Design review of the part built by this model. Coordinates are the model's own, in mm. Face numbers are marked on the shaded views. A direction names the side the tool comes from. Give positions to 0.01 mm unless a question says otherwise; leave off trailing zeros. Write each loop counter-clockwise with the first axis right and the second up, starting at its lowest first coordinate (ties: lowest second). Pieces come first, ordered by that corner, then holes.
```python
from build123d import *

# Parameters (mm, degrees)
SKETCH1_W             = 23
SKETCH1_H             = 53.06
SKETCH1_R             = 1.4732
SKETCH1_H_2           = 3.175
BOSS_EXTRUDE1_DEPTH   = 3.175
BOSS_EXTRUDE2_START   = 3.175
SKETCH1_3_W           = 23
SKETCH1_3_H           = 3.175
BOSS_EXTRUDE2_DEPTH   = 9
F_8_32_TAPPED_HOLE1_D = 3.4544
FILLET1_R             = 1


with BuildPart() as part:
    # Sketch1 → Boss-Extrude1 (new body)
    # profile 1 of 2: a face of its own
    with BuildSketch(Plane.XY):
        with Locations((11.5, -26.53)):
            Rectangle(SKETCH1_W, SKETCH1_H)
        with Locations((2.5, -5.5)):
            Circle(SKETCH1_R, mode=Mode.SUBTRACT)
        with Locations((20.5, -5.5)):
            Circle(SKETCH1_R, mode=Mode.SUBTRACT)
    # profile 2 of 2: a face of its own
    with BuildSketch(Plane.XY):
        with Locations((11.5, -54.6475)):
            Rectangle(SKETCH1_W, SKETCH1_H_2)
    extrude(amount=BOSS_EXTRUDE1_DEPTH)

    # Sketch1<3> → Boss-Extrude2 (add)
    with BuildSketch(Plane.XY.offset(BOSS_EXTRUDE2_START)):
        with Locations((11.5, -54.6475)):
            Rectangle(SKETCH1_3_W, SKETCH1_3_H)
    extrude(amount=BOSS_EXTRUDE2_DEPTH)

    # #8-32 Tapped Hole1 (through all)
    with Locations(Plane(origin=(11.5, -53.06, 8.175), x_dir=(0, 0, 1), z_dir=(0, 1, 0))):
        with Locations((0, 0)):
            Hole(F_8_32_TAPPED_HOLE1_D / 2)

    # Fillet1
    fillet1_edges = [part.edges().sort_by_distance(p)[0] for p in [
        (0, 0, 1.5875),
        (23, 0, 1.5875),
        (0, -54.6475, 12.175),
        (11.5, -53.06, 3.175),
        (23, -54.6475, 12.175),
        (11.5, -56.235, 0),
    ]]
    fillet(fillet1_edges, radius=FILLET1_R)


solid = part.part
```
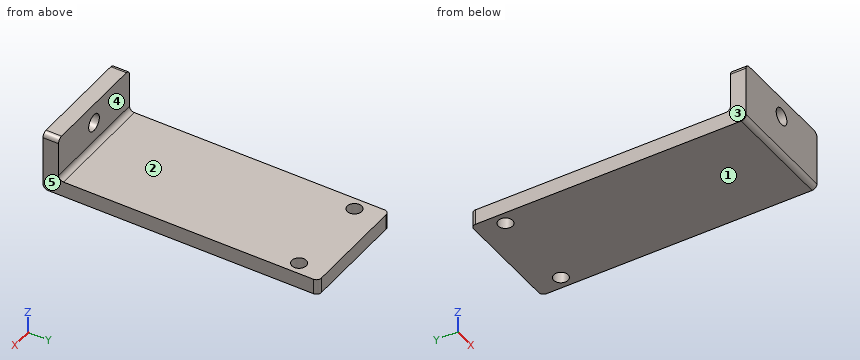
(1) To check wall thickness, follow L1, parallel to Y at x = 20.5, z = 0.9; L2, parallel to Z at x = 9.5, y = -17 (3 decimals); L3, parallel to Y at x = 4.25, z = 7.5 (3 decimals). State the ranges of each line that lie inside material, in increasing order.
Resolved:
L1: y = -56.23 to -6.97, -4.03 to 0
L2: z = 0 to 3.175
L3: y = -56.235 to -53.06
(2) Consider section A-A, the plane x = 2.5. Give the boundary of the cut face in (y, z) (3 decimals).
Resolved:
outline: (-56.235, 1) arc R1 ccw to (-55.235, 0) - (-6.973, 0) - (-6.973, 3.175) - (-52.06, 3.175) arc R1 cw to (-53.06, 4.175) - (-53.06, 12.175) - (-56.235, 12.175) - close; (-4.027, 0) - (0, 0) - (0, 3.175) - (-4.027, 3.175) - close
(3) Consider section B-B, the plane y = -5.5. Give the boundary of the cut face in (x, z) (3 decimals), then the cut area to 3 significant figures.
Resolved:
outline: (0, 0) - (1.027, 0) - (1.027, 3.175) - (0, 3.175) - close; (3.973, 0) - (19.027, 0) - (19.027, 3.175) - (3.973, 3.175) - close; (21.973, 0) - (23, 0) - (23, 3.175) - (21.973, 3.175) - close
area: 54.3 mm2
(4) Consider section D-D, the plane x = 14. Give the boundary of the cut face in (y, z) (3 decimals), then the cut area to 3 significant figures.
Resolved:
outline: (-56.235, 1) arc R1 ccw to (-55.235, 0) - (0, 0) - (0, 3.175) - (-52.06, 3.175) arc R1 cw to (-53.06, 4.175) - (-53.06, 12.175) - (-56.235, 12.175) - close
area: 207 mm2
(5) Mouldability with a two-part tool opening along Z and no side actions: class the marked faces 1, 2 and 3 as pulls with the +Z half, pulls with the -Z half, needs draft (parallel to the pull), parting line crosses it, or undercut.
Resolved:
face 1: pulls with the -Z half
face 2: pulls with the +Z half
face 3: needs draft
(6) Clearance check with flat-ended pins moving along their axes: P1, Ø1, axis at y = -23.5, z = 5, coming from the -X side; P2, Ø3, axis at x = 8.5, y = -14.5, coming from the +Z side (3 decimals). State where each tip first meets the part, or that it passes through.
Resolved:
P1: passes through
P2: stops at z = 3.175
(7) Consider section C-C, the plane z = 8. Give the boundary of the cut face in (x, y) (3 decimals), then the cut area to 3 significant figures.
Resolved:
outline: (0, -56.235) - (9.782, -56.235) - (9.782, -53.06) - (0, -53.06) - close; (13.218, -56.235) - (23, -56.235) - (23, -53.06) - (13.218, -53.06) - close
area: 62.1 mm2
(8) Tool access review of the marked faces 4 and 5: name each direction out of +Z, -Z, +X, -X, +Y, -Y from which nothing blocks a thin tool from reaching the whole face with its end or side.
Resolved:
face 4: +Z, +X, -X, +Y
face 5: +Z, -Z, +X, +Y, -Y
